from build123d import *

# Parameters (mm, degrees)
F1_DEPTH = 12.7


with BuildPart() as f1:
    # F0 (on Front) → F1 (new body)
    with BuildSketch(Plane.XZ):
        with BuildLine():
            Line((-9.130059, 101.6), (-90.936985, 101.6))
            Line((-90.936985, 101.6), (-90.936985, -25.4))
            Line((-90.936985, -25.4), (97.104346, -25.4))
            Line((97.104346, -25.4), (97.104346, 101.6))
            Line((97.104346, 101.6), (81.229346, 101.6))
            Line((81.229346, 101.6), (81.229346, 0))
            Line((81.229346, 0), (59.258346, 0))
            Line((59.258346, 0), (59.258346, -13.884136))
            Line((59.258346, -13.884136), (52.471939, -21.478448))
            Line((52.471939, -21.478448), (-13.737017, -21.478448))
            Line((-13.737017, -21.478448), (-48.406098, 0))
            ThreePointArc((-48.406098, 0), (-40.136985, 52.112136), (-31.867873, 0))
            Line((-31.867873, 0), (-13.737017, -10.196643))
            Line((-13.737017, -10.196643), (46.558346, -10.196643))
            Line((46.558346, -10.196643), (46.558346, 0))
            Line((46.558346, 0), (-9.130059, 0))
            Line((-9.130059, 0), (-9.130059, 101.6))
        make_face()
    extrude(amount=F1_DEPTH)


solid = f1.part
Model file for the job. Use its own axes, mm. A direction names the side the tool comes from. Give positions to 0.01 mm unless a question says otherwise; leave off trailing zeros. Order: outer loops, then holes, each group sorted by start corner. A loop starts at its lowest first (then second) coordinate and runs counter-clockwise, first axis right, second up. Notation, with made-up numbers: (44.5, 21.5) -> (84.5, 21.5) arc R14 ccw to (84.5, 46.5) -> close; hole circle Ø10 at (1, 22.25). An arc over 180 degrees is marked (long way). Use CSV: the item, a comma, the result in double quotes.
1. Drop flat-ended pins along their axis: pin 1 (4 mm diameter, centred on x = -7, z = 80, fed in from -Y); pin 2 (12 mm diameter, centred on x = -51.5, z = -7, fed in from +Y); pin 3 (6 mm diameter, centred on x = 55.5, y = -11, fed in from +Z). Give the stop position or say it passes through.
Outcome:
pin 1,"through"
pin 2,"y = 0"
pin 3,"z = -14.73"
2. Band-saw the part on D-D, the plane z = 25.4. Give the cut face in (x, y).
Outcome:
outline,"(-90.94, -12.7) -> (-66.85, -12.7) -> (-66.85, 0) -> (-90.94, 0) -> close; (-13.42, -12.7) -> (-9.13, -12.7) -> (-9.13, 0) -> (-13.42, 0) -> close; (81.23, -12.7) -> (97.1, -12.7) -> (97.1, 0) -> (81.23, 0) -> close"
3. Band-saw the part on C-C, the plane y = -6.25. Give the cut face in (x, z), then the cut area to 3 significant figures.
Outcome:
outline,"(-90.94, -25.4) -> (97.1, -25.4) -> (97.1, 101.6) -> (81.23, 101.6) -> (81.23, 0) -> (59.26, 0) -> (59.26, -13.88) -> (52.47, -21.48) -> (-13.74, -21.48) -> (-48.41, 0) arc R26.71 cw (long way) to (-31.87, 0) -> (-13.74, -10.2) -> (46.56, -10.2) -> (46.56, 0) -> (-9.13, 0) -> (-9.13, 101.6) -> (-90.94, 101.6) -> close"
area,"11,300 mm²"
4. Band-saw the part on B-B, the plane z = 60. Give the cut face in (x, y).
Outcome:
outline,"(-90.94, -12.7) -> (-9.13, -12.7) -> (-9.13, 0) -> (-90.94, 0) -> close; (81.23, -12.7) -> (97.1, -12.7) -> (97.1, 0) -> (81.23, 0) -> close"
5. Band-saw the part on A-A, the plane x = 21.5. Give the cut face in (y, z).
Outcome:
outline,"(-12.7, -25.4) -> (0, -25.4) -> (0, -21.48) -> (-12.7, -21.48) -> close; (-12.7, -10.2) -> (0, -10.2) -> (0, 0) -> (-12.7, 0) -> close"
6. Mould opens along Z. For faces 1 (the flat face through (55.91, -6.26, -17.63)), 2 (the flat face through (46.558, -6, -5)), 3 (the flat face through (-22.929, -6.261, -5.027)) say: +Z half, -Z half, draft (parallel to the pull), parting line (faces both ways), or undercut.
Outcome:
face 1,"+Z half"
face 2,"draft"
face 3,"undercut"
7. 3-axis set-ups, long thin cutter, end or side, ignore diameter. For faces 4 (the flat face through (-19, 0, 53)), 5 (the flat face through (16, -6, -10.197)), 6 (the flat face through (81.229, -6, 52)): which of +Z, -Z, +X, -X, +Y, -Y reach the whole face in a straight line?
Outcome:
face 4,"+Z, -Z, +X, -X, +Y"
face 5,"+Y, -Y"
face 6,"+Z, +Y, -Y"
8. Drill centre lines: line 1 along X through (y, z) = (-3.75, 25.4); line 2 along X through (y, z) = (-3.5, 37); line 3 along Z through (x, y) = (-18, -0.75). Where is each one in solid material? Low to high. Write a range as from..to.
Outcome:
line 1,"-90.94..-66.85, -13.42..-9.13, 81.23..97.1"
line 2,"-90.94..-64.2, -16.08..-9.13, 81.23..97.1"
line 3,"-25.4..-18.84, -7.8..10.45, 40.35..101.6"
